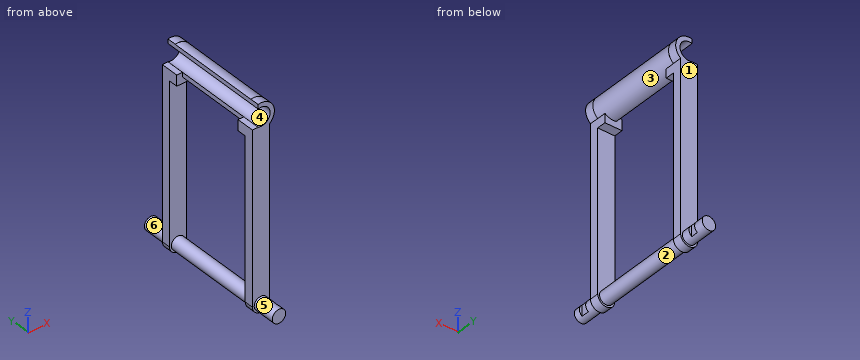
```python
from build123d import *

# Parameters (mm, degrees)
EXTRUDE_1_DEPTH     = 2
SKETCH_2_R          = 3
EXTRUDE_2_DEPTH     = 10.5
SKETCH_3_R          = 2.05
CUT_EXTRUDE_1_DEPTH = 12.5
EXTRUDE_3_DEPTH     = 2
SKETCH_5_R          = 3
SKETCH_5_R_2        = 2.05
EXTRUDE_4_DEPTH     = 2
SKETCH_8_W          = 2.95616439
SKETCH_8_H          = 6.387063899
CUT_EXTRUDE_3_DEPTH = 12.5
SKETCH_9_W          = 1.27668382
SKETCH_9_H          = 4
EXTRUDE_5_DEPTH     = 1
SKETCH_10_R         = 1.5
EXTRUDE_6_DEPTH     = 10.5
MIRROR_START        = 23
MIRROR_11_DEPTH     = 2
SKETCH_11_R         = 1.5
EXTRUDE_7_DEPTH     = 18
EXTRUDE_START       = 5
SKETCH_12_R         = 1.5
EXTRUDE_8_DEPTH     = 5
SKETCH_13_W         = 5.222026014
SKETCH_13_H         = 1.730667712
SKETCH_13_H_2       = 1.553374839
CUT_EXTRUDE_4_DEPTH = 1


# Read off the part's stored shape, not the designer's step: 镜向11
with BuildPart() as part:
    # 草图1 → 凸台-拉伸1 (new body)
    with BuildSketch(Plane(origin=(0, 0, 0), x_dir=(1, 0, 0), z_dir=(0, 1, 0))):
        with BuildLine():
            Line((1.9, 0), (1.9, -40.018240839))
            ThreePointArc((1.9, -40.018240839), (0, -41.918240839), (-1.9, -40.018240839))
            Line((-1.9, -40.018240839), (-1.9, 0))
            ThreePointArc((-1.9, 0), (0, 1.9), (1.9, 0))
        make_face()
    extrude(amount=EXTRUDE_1_DEPTH)

    # 草图2 → 凸台-拉伸2 (add)
    with BuildSketch(Plane(origin=(0, 2, 0), x_dir=(1, 0, 0), z_dir=(0, 1, 0))):
        with Locations(Location((0, -39.871991717, 0), (0, 0, 129.296480239))):
            Circle(SKETCH_2_R)
    extrude_2 = extrude(amount=EXTRUDE_2_DEPTH)

    # 草图3 → 切除-拉伸1 (cut)
    with BuildSketch(Plane(origin=(0, 12.5, 0), x_dir=(1, 0, 0), z_dir=(0, 1, 0))):
        with Locations(Location((0, -39.903679128, 0), (0, 0, 270))):
            Circle(SKETCH_3_R)
    cut_extrude_1 = extrude(amount=-CUT_EXTRUDE_1_DEPTH, mode=Mode.SUBTRACT)

    # 草图4 → 凸台-拉伸3 (add)
    with BuildSketch(Plane(origin=(0, 2, 0), x_dir=(1, 0, 0), z_dir=(0, 1, 0))):
        with BuildLine():
            Line((-1.9, -35.550354364), (-1.9, -37.550354364))
            ThreePointArc((-1.9, -37.550354364), (-1.008733845, -37.046667659), (0, -36.871991717))
            ThreePointArc((0, -36.871991717), (1.008733845, -37.046667659), (1.9, -37.550354364))
            Line((1.9, -37.550354364), (1.9, -35.550354364))
            Line((1.9, -35.550354364), (-1.9, -35.550354364))
        make_face()
    extrude_3 = extrude(amount=EXTRUDE_3_DEPTH)

    # 草图5 → 凸台-拉伸4 (add)
    with BuildSketch(Plane.XZ.offset(-2)):
        with Locations((0, 39.903679128)):
            Circle(SKETCH_5_R)
        with Locations(Location((0, 39.903679128, 0), (0, 0, 90))):
            Circle(SKETCH_5_R_2, mode=Mode.SUBTRACT)
    extrude_4 = extrude(amount=EXTRUDE_4_DEPTH)

    # 草图8 → 切除-拉伸3 (cut)
    with BuildSketch(Plane(origin=(0, 12.5, 0), x_dir=(1, 0, 0), z_dir=(0, 1, 0))):
        with Locations((-2.101398375, -40.130991858)):
            Rectangle(SKETCH_8_W, SKETCH_8_H)
    cut_extrude_3 = extrude(amount=-CUT_EXTRUDE_3_DEPTH, mode=Mode.SUBTRACT)

    # 草图9 → 凸台-拉伸5 (add)
    with BuildSketch(Plane.XY.offset(36.937459908)):
        with Locations((-1.26165809, 2)):
            Rectangle(SKETCH_9_W, SKETCH_9_H)
    extrude_5 = extrude(amount=EXTRUDE_5_DEPTH)

    # 草图10 → 凸台-拉伸6 (add)
    with BuildSketch(Plane(origin=(0, 2, 0), x_dir=(1, 0, 0), z_dir=(0, 1, 0))):
        with Locations(Location((0, 0, 0), (0, 0, 90))):
            Circle(SKETCH_10_R)
    extrude(amount=EXTRUDE_6_DEPTH)

    # 镜向10: 凸台-拉伸2, 切除-拉伸1, 凸台-拉伸3, 凸台-拉伸4, 切除-拉伸3, 凸台-拉伸5 across plane
    add(extrude_2.mirror(Plane.ZX.offset(12.5)))
    add(cut_extrude_1.mirror(Plane.ZX.offset(12.5)), mode=Mode.SUBTRACT)
    add(extrude_3.mirror(Plane.ZX.offset(12.5)))
    add(extrude_4.mirror(Plane.ZX.offset(12.5)))
    add(cut_extrude_3.mirror(Plane.ZX.offset(12.5)), mode=Mode.SUBTRACT)
    add(extrude_5.mirror(Plane.ZX.offset(12.5)))

    # 镜向11 outline → 镜向11 (add)
    with BuildSketch(Plane(origin=(0, 0, 0), x_dir=(1, 0, 0), z_dir=(0, 1, 0)).offset(MIRROR_START)):
        with BuildLine():
            ThreePointArc((1.9, 0), (0, 1.9), (-1.9, 0))
            Line((-1.9, 0), (-1.9, -36.937459908))
            Line((-1.9, -36.937459908), (-0.62331618, -36.937459908))
            Line((-0.62331618, -36.937459908), (-0.62331618, -36.969147319))
            ThreePointArc((-0.62331618, -36.969147319), (0.708089188, -36.988441625), (1.9, -37.582041775))
            Line((1.9, -37.582041775), (1.9, 0))
        make_face()
    extrude(amount=MIRROR_11_DEPTH)

    # 草图11 → 凸台-拉伸7 (add)
    with BuildSketch(Plane(origin=(0, 12.5, 0), x_dir=(1, 0, 0), z_dir=(0, 1, 0))):
        with Locations(Location((0, 0, 0), (0, 0, 90))):
            Circle(SKETCH_11_R)
    extrude(amount=EXTRUDE_7_DEPTH)

    # 草图12 → 凸台-拉伸8 (add)
    with BuildSketch(Plane.XZ.offset(EXTRUDE_START)):
        with Locations(Location((0, 0, 0), (0, 0, 270))):
            Circle(SKETCH_12_R)
    extrude(amount=-EXTRUDE_8_DEPTH)

    # 草图13 → 切除-拉伸4 (cut)
    with BuildSketch(Plane(origin=(1.9, 0, 0), x_dir=(0, 0, -1), z_dir=(1, 0, 0))):
        with Locations((0.263368909, -2.718253364)):
            Rectangle(SKETCH_13_W, SKETCH_13_H)
        with Locations((0.263368909, 27.61617656)):
            Rectangle(SKETCH_13_W, SKETCH_13_H_2)
    extrude(amount=-CUT_EXTRUDE_4_DEPTH, mode=Mode.SUBTRACT)


solid = part.part
```
For this review, take the finished solid that the model builds, in its own axes (mm). Face numbers are marked on the shaded views. A direction names the side the tool comes from. Give positions to 0.01 mm unless a question says otherwise; leave off trailing zeros. Write each loop counter-clockwise with the first axis right and the second up, starting at its lowest first coordinate (ties: lowest second). Pieces come first, ordered by that corner, then holes. Notation, with made-up numbers: M 52,59.5 L 70,59.5 A7 ccw 70,64.5 Z; hole C 12.5,19.25 d10. An arc over 180 degrees is marked long. Answer as CSV lines item,"result".
1. For the marked faces 5 and 6, list the 3-axis set-ups (+Z, -Z, +X, -X, +Y, -Y) from which the entire face can be reached by the end or side of a thin tool; tool diameter is ignored.
Findings:
face 5,"-Y"
face 6,"+Y"
2. Consider section A-A, the plane x = 0. Count the separate pieces of the cut face and the enclosed holes in it, then the cut area to 3 significant figures.
Findings:
separate pieces,"2"
enclosed holes,"1"
area,"303 mm2"
3. Consider section C-C, the plane y = 7.5. Write out the cut boundary in (x, z).
Findings:
outline,"C 0,0 d3; M -0.62,36.94 A3 ccw long -0.62,42.81 L -0.62,41.86 A2.05 cw long -0.62,37.95 Z"
4. Consider section B-B, the plane z = 2. Write out the cut boundary in (x, y).
Findings:
outline,"M -1.9,0 L 1.9,0 L 1.9,2 L -1.9,2 Z; M -1.9,23 L 1.9,23 L 1.9,25 L -1.9,25 Z"
5. Consider section D-D, the plane y = 25.5. Write out the cut boundary in (x, z), then the cut area to 3 significant figures.
Findings:
outline,"C 0,0 d3"
area,"7.07 mm2"
6. Wall thickness on line 1 (Y direction, x = -1.7, z = 35); line 2 (Y direction, x = 0.55, z = 36); line 3 (Z direction, x = -0.4, y = 8.5): over which ranges is each line inside the solid? List them lowest first.
Findings:
line 1,"y = 0 to 2, 23 to 25"
line 2,"y = 0 to 4, 21 to 25"
line 3,"z = -1.45 to 1.45, 36.9 to 37.89, 41.91 to 42.85"
7. Draft analysis for pull direction Y (two halves, no side actions). For the marked faces 1, 2, 3 and 4, state which applies: +Y half, -Y half, draft (parallel to the pull), parting line (faces both ways), or undercut.
Findings:
face 1,"+Y half"
face 2,"undercut"
face 3,"undercut"
face 4,"draft"
8. For pin 1 (1 mm diameter, centred on x = 1, y = 22, fed in from -Z); pin 2 (1.7 mm diameter, centred on y = 27.5, z = 0, fed in from +X); pin 3 (1.9 mm diameter, centred on x = -0.5, z = 36.5, fed in from +Y); pin 4 (4 mm diameter, centred on y = 3, z = 28, fed in from -X), all flat-tipped, find the tip position at first contact; note any pin that passes through.
Findings:
pin 1,"stops at z = -1.41"
pin 2,"stops at x = 1.5"
pin 3,"stops at y = 25"
pin 4,"stops at x = -1.9"
